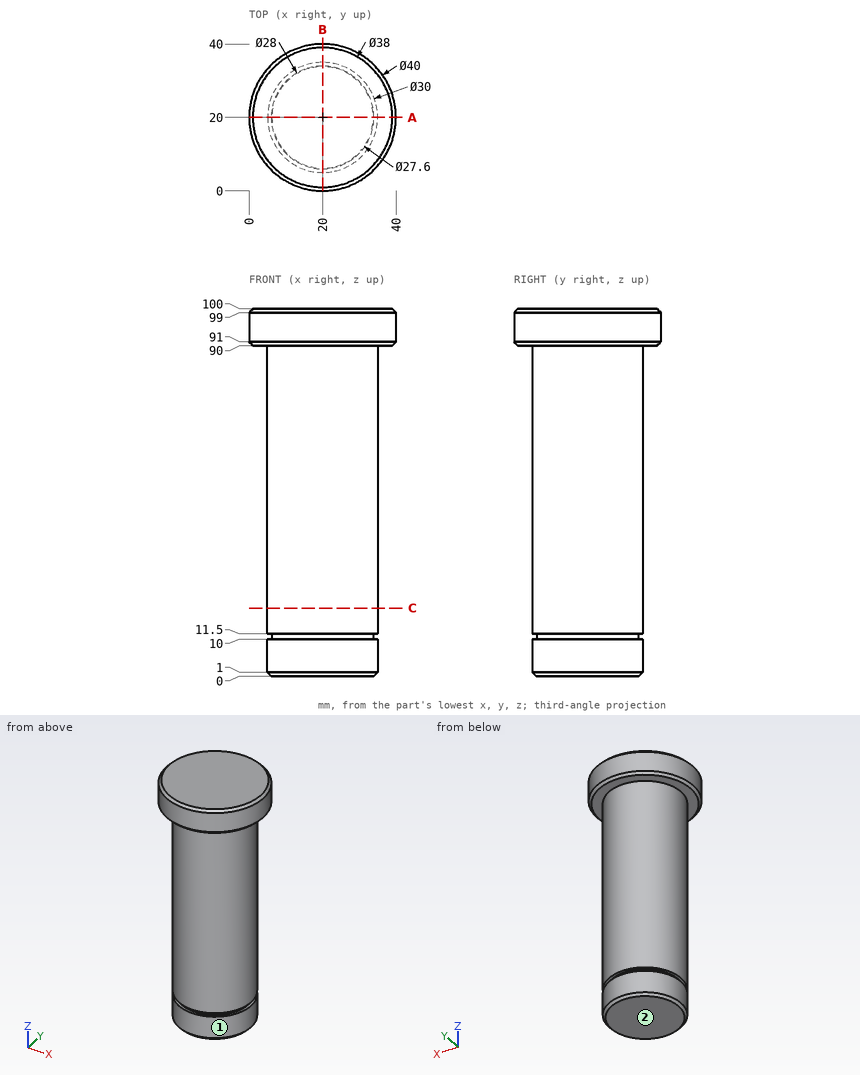
Geometry check sheet. Reference: drawing and pictorial views, mm from the part's lowest x, y, z. A direction names the side the tool comes from. Give positions to 0.01 mm unless a question says otherwise; leave off trailing zeros. Loops run counter-clockwise (first coordinate to the right, second up) from the corner with the lowest first, then second, coordinate; pieces in that order, holes last. Notation, with made-up numbers: M -19,86.25 L -2,86.25 A7 ccw -2,96.25 Z; hole C -28.75,16 d9. An arc over 180 degrees is marked long. Use a Markdown table: item, result. Add a question column.
Q1. Sectioned sample at A-A, the plane y = 20. Record the cut outline in (x, z).
Q2. Sectioned sample at C-C, the plane z = 18.5. Record the cut outline in (x, y).
Q3. Scan lines: line 1 along Z through (x, y) = (13.5, 2.5); line 2 along Y through (x, z) = (19.5, 21); line 3 along Z through (x, y) = (8, 12.5). Record each from-to range of solid material in increasing order. Write a range as [from, to].
Q4. Go/stop test with flat-tipped pins: pin 1 (3 mm diameter, centred on x = 24, z = 50, fed in from -Y); pin 2 (4 mm diameter, centred on y = 7.5, z = 75, fed in from +X); pin 3 (6 mm diameter, centred on y = 27, z = 78.5, fed in from -X). Record where each tip stops, or that it passes through.
Q5. Tool access check on the marked faces 1 and 2. Record the directions out of +Z, -Z, +X, -X, +Y, -Y that give a thin tool (end or side, any length) a straight path to the whole face; none if there is none.
Verdict:
| question | item | result |
|---|---|---|
| 1 | outline | M 0,91 L 1,90 L 5,90 L 5,11.5 L 6.2,11.5 L 6.2,10 L 5,10 L 5,1 L 6,0 L 34,0 L 35,1 L 35,10 L 33.8,10 L 33.8,11.5 L 35,11.5 L 35,90 L 39,90 L 40,91 L 40,99 L 39,100 L 1,100 L 0,99 Z |
| 2 | outline | C 20,20 d30 |
| 3 | line 1 | [90, 100] |
| 3 | line 2 | [5.01, 34.99] |
| 3 | line 3 | [0.15, 10], [11.5, 100] |
| 4 | pin 1 | y = 5.21 |
| 4 | pin 2 | x = 30.71 |
| 4 | pin 3 | x = 5.54 |
| 5 | face 1 | -Z |
| 5 | face 2 | -Z, +X, -X, +Y, -Y |
